from build123d import *

# Parameters (mm, degrees)
F0_R     = 5
F1_DEPTH = 22
F0_R_2   = 8
F2_DEPTH = 10
F4_DEPTH = 8
F5_R     = 0.2
F6_R     = 1


# Not quite as in the source:
# - a feature names something its author has since deleted; it is built from what else it names


with BuildPart() as f1:
    # F0 (on Front) → F1 (new body)
    with BuildSketch(Plane.XZ):
        Circle(F0_R)
    extrude(amount=F1_DEPTH)

    # F0 (on Front) → F2 (join)
    with BuildSketch(Plane.XZ):
        Circle(F0_R_2)
        Circle(F0_R, mode=Mode.SUBTRACT)
        Circle(F0_R)
    extrude(amount=-F2_DEPTH)

    # F3 (on face) → F4 (cut)
    with BuildSketch(Plane(origin=(0, 10, 0), x_dir=(-1, 0, 0), z_dir=(0, 1, 0))):
        Polygon((-2.3094010768, -4), (2.3094010768, -4), (4.6188021535, 0), (2.3094010768, 4), (-2.3094010768, 4), (-4.6188021535, 0), align=None)
    extrude(amount=-F4_DEPTH, mode=Mode.SUBTRACT)

    # F5
    f5_edges = [f1.edges().sort_by_distance(p)[0] for p in [
        (-3.464102, 2, 2),
        (3.464102, 2, -2),
        (0, 2, 4),
        (0, 10, -4),
        (-3.464102, 2, -2),
        (0, 2, -4),
        (3.464102, 10, 2),
        (3.464102, 2, 2),
        (-3.464102, 10, -2),
        (-3.464102, 10, 2),
        (-8, 10, 0),
        (0, 10, 4),
        (3.464102, 10, -2),
        (-8, 0, 0),
    ]]
    fillet(f5_edges, radius=F5_R)

    # F6
    f6_edges = [f1.edges().sort_by_distance(p)[0] for p in [
        (-5, -22, 0),
    ]]
    fillet(f6_edges, radius=F6_R)


solid = f1.part
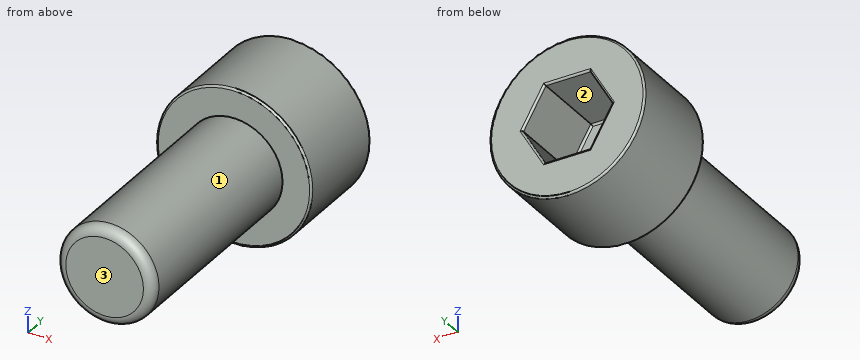
CAD build for the part. Positions are in the model's coordinates, mm. Face numbers are marked on the shaded views. A direction names the side the tool comes from. Coordinates: 2 decimals unless noted, no trailing zeros. Loops run counter-clockwise (first coordinate to the right, second up) from the corner with the lowest first, then second, coordinate; pieces in that order, holes last. Notation, with made-up numbers: (-39, 56) - (-10, 56) arc R32 cw to (-10, 95) - close; hole circle Ø3 at (-27, 84). An arc over 180 degrees is marked (long way). Write item = value, one per line. Start each with the question number.
Q1. Drill centre lines: L1, parallel to Z at x = -0.25, y = 7; L2, parallel to Z at x = -3.25, y = 8; L3, parallel to X at y = 7, z = -2.5. Where is each one in solid material? Low to high.
Q2. Cut at B-B, the plane y = -17. List the corners of the cut face in (x, z).
Q3. Cut at A-A, the plane x = 0. List the corners of the cut face in (y, z), then the cut area to 3 significant figures.
Q4. Flat gauge pins, fed straight in: pin 1 Ø4 at (y, z) = (-15, -3) entering from +X; pin 2 Ø1 at (y, z) = (-8, -3.5) entering from +X; pin 3 Ø2 at (x, y) = (4, -0.5) entering from -Z; pin 4 Ø3.5 at (x, y) = (0.5, 5) entering from -Z. Where does each tip first touch, or does it go through?
Q5. Which spindle directions (+Z, -Z, +X, -X, +Y, -Y) get a long thin tool onto all of the face, cutting with end or side? Do the marked faces 1, 2 and 3. Say none if no direction does.
Computed:
q1.L1 = -8 to -4, 4 to 8
q1.L2 = -7.31 to -2.37, 2.37 to 7.31
q1.L3 = -7.6 to -3.18, 3.18 to 7.6
q2.outline = circle Ø10 at (0, 0)
q3.outline = (-22, -4) arc R1 ccw to (-21, -5) - (0, -5) - (0, -7.8) arc R0.2 ccw to (0.2, -8) - (9.8, -8) arc R0.2 ccw to (10, -7.8) - (10, -4.2) arc R0.2 ccw to (9.8, -4) - (2.2, -4) arc R0.2 cw to (2, -3.8) - (2, 3.8) arc R0.2 cw to (2.2, 4) - (9.8, 4) arc R0.2 ccw to (10, 4.2) - (10, 7.8) arc R0.2 ccw to (9.8, 8) - (0.2, 8) arc R0.2 ccw to (0, 7.8) - (0, 5) - (-21, 5) arc R1 ccw to (-22, 4) - close
q3.area = 316 mm²
q4.pin_1 = 4.9
q4.pin_2 = 4
q4.pin_3 = -7.31
q4.pin_4 = -8
q5.face_1 = -Y
q5.face_2 = +Y
q5.face_3 = +Z, -Z, +X, -X, -Y
